Part model, mm, in its own coordinate system. Face numbers are marked on the shaded views. Round coordinates to 2 decimals unless told otherwise and drop trailing zeros. Write each loop counter-clockwise with the first axis right and the second up, starting at its lowest first coordinate (ties: lowest second). Pieces come first, ordered by that corner, then holes. Notation, with made-up numbers: (-27, 66) -> (7, 66) arc R35 ccw to (7, 103) -> close; hole circle Ø8 at (10.25, -19). An arc over 180 degrees is marked (long way). Use CSV: the item, a comma, the result in double quotes. Start each with the question number.
(1) Drop flat-ended pins along their axis: pin 1 (12 mm diameter, centred on x = -18, y = 16, fed in from -Z); pin 2 (10 mm diameter, centred on x = -12.5, y = -16.5, fed in from -Z); pin 3 (1.9 mm diameter, centred on x = 21.5, y = 21.5, fed in from -Z); pin 4 (3 mm diameter, centred on x = 10.5, z = 15.5, fed in from -Y). Give the stop position or say it passes through.
(2) Saw through at C-C (z = 18.75). Give the cut face in (x, y), plus the area to 3 significant figures.
(3) Two-plate mould, pull along Y, no slides. Class the marked faces 1, 2 and 3: released by +Y, released by -Y, zero draft, split by the parting line, or undercut.
(4) Saw through at B-B (z = 7.25). Give the cut face in (x, y), plus the area to 3 significant figures.
(5) Probe line 1 (Y direction, x = -21.5, z = 21); line 2 (Z direction, x = 15.5, y = -6.5); line 3 (Y direction, x = 0, z = 13.75). List the from-to ranges inside material, lowest first. Write a range as [from, to].
(6) Saw through at A-A (y = 0). Count the separate pieces of the cut face and the enclosed holes in it, plus the area to 3 significant figures.
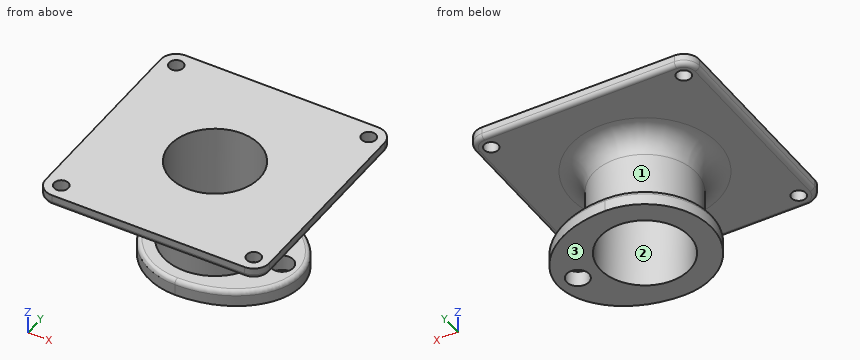
```python
from build123d import *

# Parameters (mm, degrees)
BOSS_EXTRUDE1_OUTLINE_R   = 10
BOSS_EXTRUDE1_OUTLINE_R_2 = 2.5
BOSS_EXTRUDE1_DEPTH       = 3.5
SKETCH1_3_R               = 11.5
SKETCH1_3_R_2             = 10
BOSS_EXTRUDE2_DEPTH       = 20
SKETCH2_W                 = 50
SKETCH2_H                 = 50
SKETCH2_R                 = 1.6
SKETCH2_R_2               = 11.5
SKETCH2_R_3               = 10
BOSS_EXTRUDE3_DEPTH       = 2.5
FILLET1_R                 = 3.5
FILLET2_R                 = 5
FILLET3_R                 = 1


# Read off the part's stored shape, not the designer's step: Boss-Extrude1
with BuildPart() as part:
    # Boss-Extrude1 outline → Boss-Extrude1 (new body)
    with BuildSketch(Plane.XY):
        with BuildLine():
            ThreePointArc((0, 15), (-15, 0), (0, -15))
            add(Edge.make_bspline(
                [(0, -15), (11.666666667, -15), (19.5, -7.666459565), (19.5, 7.333540435), (11.666666667, 15), (0, 15)],
                knots=[0, 0, 0, 0, 0.511097304, 0.511097304, 1, 1, 1, 1], degree=3))
        make_face()
        Circle(BOSS_EXTRUDE1_OUTLINE_R, mode=Mode.SUBTRACT)
        with Locations((15, 0)):
            Circle(BOSS_EXTRUDE1_OUTLINE_R_2, mode=Mode.SUBTRACT)
    extrude(amount=BOSS_EXTRUDE1_DEPTH)

    # Sketch1<3> → Boss-Extrude2 (add)
    with BuildSketch(Plane.XY):
        Circle(SKETCH1_3_R)
        Circle(SKETCH1_3_R_2, mode=Mode.SUBTRACT)
    extrude(amount=BOSS_EXTRUDE2_DEPTH)

    # Sketch2 → Boss-Extrude3 (add)
    # profile 1 of 2: a face of its own
    with BuildSketch(Plane.XY.offset(20)):
        Rectangle(SKETCH2_W, SKETCH2_H)
        with Locations((21.5, 21.5)):
            Circle(SKETCH2_R, mode=Mode.SUBTRACT)
        with Locations((21.5, -21.5)):
            Circle(SKETCH2_R, mode=Mode.SUBTRACT)
        with Locations((-21.5, -21.5)):
            Circle(SKETCH2_R, mode=Mode.SUBTRACT)
        with Locations((-21.5, 21.5)):
            Circle(SKETCH2_R, mode=Mode.SUBTRACT)
        Circle(SKETCH2_R_2, mode=Mode.SUBTRACT)
    # profile 2 of 2: a face of its own
    with BuildSketch(Plane.XY.offset(20)):
        Circle(SKETCH2_R_2)
        Circle(SKETCH2_R_3, mode=Mode.SUBTRACT)
    extrude(amount=BOSS_EXTRUDE3_DEPTH)

    # Fillet1
    fillet1_edges = [part.edges().sort_by_distance(p)[0] for p in [
        (25, -25, 21.25),
        (25, 25, 21.25),
        (-25, 25, 21.25),
        (-25, -25, 21.25),
    ]]
    fillet(fillet1_edges, radius=FILLET1_R)

    # Fillet2
    fillet2_edges = [part.edges().sort_by_distance(p)[0] for p in [
        (-11.5, 0, 20),
    ]]
    fillet(fillet2_edges, radius=FILLET2_R)

    # Fillet3
    fillet3_edges = [part.edges().sort_by_distance(p)[0] for p in [
        (-15, 0, 3.5),
        (25, 0, 20),
        (0, -25, 20),
        (-25, 0, 20),
        (0, 25, 20),
        (23.974873734, 23.974873734, 20),
        (-23.974873734, 23.974873734, 20),
        (-23.974873734, -23.974873734, 20),
        (23.974873734, -23.974873734, 20),
        (10, 0, 11.25),
    ]]
    fillet(fillet3_edges, radius=FILLET3_R)


solid = part.part
```
Answers:
1,pin 1,"stops at z = 20"
1,pin 2,"stops at z = 19.94"
1,pin 3,"passes through"
1,pin 4,"stops at y = -7.22"
2,outline,"circle Ø26.39 at (0, 0); hole circle Ø20 at (0, 0)"
2,area,"233 mm²"
3,face 1,"split by the parting line"
3,face 2,"undercut"
3,face 3,"zero draft"
4,outline,"circle Ø23 at (0, 0); hole circle Ø20 at (0, 0)"
4,area,"101 mm²"
5,line 1,"y = [-25, -23.1], [-19.9, 19.9], [23.1, 25]"
5,line 2,"z = [0, 3.5], [20, 22.5]"
5,line 3,"y = [-11.5, -10], [10, 11.5]"
6,separate pieces,"3"
6,enclosed holes,"0"
6,area,"168 mm²"
